```python
from build123d import *

# Parameters (mm, degrees)
BASE_SKETCH_R = 0.5969
BASE_DEPTH    = 0.889


with BuildPart() as part:
    # Base Sketch → Base (new body)
    with BuildSketch(Plane.XY):
        with BuildLine():
            Line((-2.321834428, -4.191), (-3.275039722, -5.842))
            ThreePointArc((-3.275039722, -5.842), (-3.775058057, -6.206035718), (-4.38041724, -6.079226415))
            ThreePointArc((-4.38041724, -6.079226415), (0, 7.493), (4.38041724, -6.079226415))
            ThreePointArc((4.38041724, -6.079226415), (3.775058057, -6.206035718), (3.275039722, -5.842))
            Line((3.275039722, -5.842), (2.321834428, -4.191))
            ThreePointArc((2.321834428, -4.191), (2.321834428, -3.429), (2.981745785, -3.048))
            Line((2.981745785, -3.048), (6.018835366, -3.048))
            ThreePointArc((6.018835366, -3.048), (0, 6.2738), (-6.018835366, -3.048))
            Line((-6.018835366, -3.048), (-2.981745785, -3.048))
            ThreePointArc((-2.981745785, -3.048), (-2.321834428, -3.429), (-2.321834428, -4.191))
        make_face()
        with Locations((3.6195, -4.318)):
            Circle(BASE_SKETCH_R, mode=Mode.SUBTRACT)
        with Locations(Location((-3.6195, -4.318, 0), (0, 0, 180))):
            Circle(BASE_SKETCH_R, mode=Mode.SUBTRACT)
    extrude(amount=-BASE_DEPTH)


solid = part.part
```
Geometry: final body of the model. Coordinates: model frame, mm. A direction names the side the tool comes from. Coordinates: 2 decimals unless noted, no trailing zeros. Loops run counter-clockwise (first coordinate to the right, second up) from the corner with the lowest first, then second, coordinate; pieces in that order, holes last. Notation, with made-up numbers: (3.25, 86) -> (27.25, 86) arc R27 cw to (27.25, 111) -> close; hole circle Ø3 at (-23, -17.75). An arc over 180 degrees is marked (long way). Use a Markdown table: item, result. Add a question column.
(1) Pin query (flat end, axial travel): pin 1 Ø1.1 at (x, y) = (3.62, -4.32) entering from -Z. Return the tip coordinate at first contact, or that it passes through.
(2) Section query B-B, the plane y = 0. Return loops of the section in (x, z).
(3) Mould query, pull axis X, two halves, no side actions, for faces 4 (the flat face through (-2.7, -3.4, -0.889)), 5 (the cylindrical face through (-0.26, 7.49, -0.44)), 6 (the cylindrical face through (-2.327, -3.419, -0.438)). Classes: pulls with the +X half, pulls with the -X half, needs draft (parallel to the pull), parting line crosses it, or undercut.
(4) Section query A-A, the plane x = 4. Return loops of the section in (y, z).
(5) Line query: line 1 along X through (y, z) = (-4.25, -0.3); line 2 along X through (y, z) = (-4.75, -0.8); line 3 along Y through (x, z) = (-3.25, -0.65). Output: solid intervals per line, ascending.
(6) Section query D-D, the plane x = 0. Return loops of the section in (y, z), plus the area to 3 significant figures.
(7) Access query for faces 1 (the flat face through (-2.7, -3.4, 0)), 2 (the flat face through (-2.79, -5, -0.44)), 3 (the cylindrical face through (2.316, -3.439, -0.438)). Directions: +Z, -Z, +X, -X, +Y, -Y. A direction counts if a zero-diameter tool reaches every point of the face in a straight line with its end or side. Return the directions, or none.
(8) Section query C-C, the plane z = -0.15. Return loops of the section in (x, y), plus the area to 3 significant figures.
Answer:
| question | item | result |
|---|---|---|
| 1 | pin 1 | passes through |
| 2 | outline | (-7.49, -0.89) -> (-6.6, -0.89) -> (-6.6, 0) -> (-7.49, 0) -> close; (6.6, -0.89) -> (7.49, -0.89) -> (7.49, 0) -> (6.6, 0) -> close |
| 3 | face 4 | needs draft |
| 3 | face 5 | parting line crosses it |
| 3 | face 6 | undercut |
| 4 | outline | (-6.22, -0.89) -> (-4.78, -0.89) -> (-4.78, 0) -> (-6.22, 0) -> close; (-3.86, -0.89) -> (-3.05, -0.89) -> (-3.05, 0) -> (-3.86, 0) -> close; (4.92, -0.89) -> (6.34, -0.89) -> (6.34, 0) -> (4.92, 0) -> close |
| 5 | line 1 | x = -6.17 to -4.21, -3.03 to -2.36, 2.36 to 3.03, 4.21 to 6.17 |
| 5 | line 2 | x = -5.8 to -4.03, -3.21 to -2.64, 2.64 to 3.21, 4.03 to 5.8 |
| 5 | line 3 | y = -5.8 to -4.79, -3.85 to -3.05, 5.42 to 6.75 |
| 6 | outline | (6.27, -0.89) -> (7.49, -0.89) -> (7.49, 0) -> (6.27, 0) -> close |
| 6 | area | 1.08 mm^2 |
| 7 | face 1 | +Z, +X, -X, +Y, -Y |
| 7 | face 2 | +Z, -Z, -Y |
| 7 | face 3 | +Z, -Z |
| 8 | outline | (-6.02, -3.05) arc R6.6 cw (long way) to (6.02, -3.05) -> (2.98, -3.05) arc R0.76 ccw to (2.32, -4.19) -> (3.28, -5.84) arc R0.76 ccw to (4.38, -6.08) arc R7.49 ccw (long way) to (-4.38, -6.08) arc R0.76 ccw to (-3.28, -5.84) -> (-2.32, -4.19) arc R0.76 ccw to (-2.98, -3.05) -> close; hole circle Ø1.19 at (-3.62, -4.32); hole circle Ø1.19 at (3.62, -4.32) |
| 8 | area | 46.3 mm^2 |
